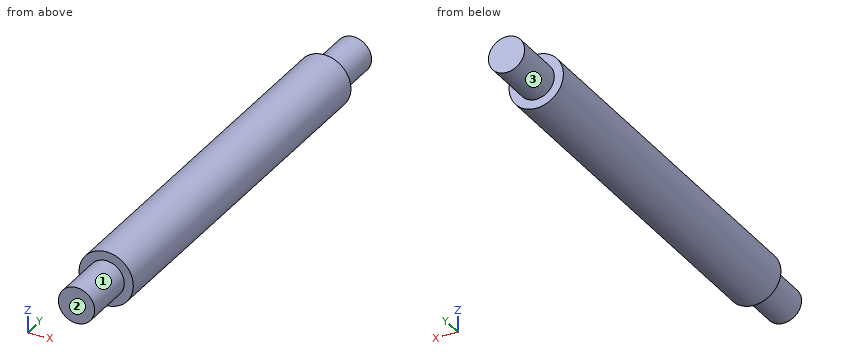
```python
from build123d import *

# Parameters (mm, degrees)
F0_R     = 4.7625
F1_DEPTH = 44.45
F2_R     = 6.35
F2_R_2   = 3.175
F3_DEPTH = 9.525
F4_R     = 6.35
F4_R_2   = 3.175
F5_DEPTH = 9.525


with BuildPart() as f1:
    # F0 (on Front) → F1 (new body, symmetric)
    with BuildSketch(Plane.XZ):
        Circle(F0_R)
    extrude(amount=F1_DEPTH, both=True)

    # F2 (on face) → F3 (cut)
    with BuildSketch(Plane.XZ.offset(44.45)):
        Circle(F2_R)
        Circle(F2_R_2, mode=Mode.SUBTRACT)
    extrude(amount=-F3_DEPTH, mode=Mode.SUBTRACT)

    # F4 (on face) → F5 (cut)
    with BuildSketch(Plane(origin=(0, 44.45, 0), x_dir=(-1, 0, 0), z_dir=(0, 1, 0))):
        Circle(F4_R)
        Circle(F4_R_2, mode=Mode.SUBTRACT)
    extrude(amount=-F5_DEPTH, mode=Mode.SUBTRACT)


solid = f1.part
```
Geometry: final body of the model. Coordinates: model frame, mm. Face numbers are marked on the shaded views. A direction names the side the tool comes from. Coordinates: 2 decimals unless noted, no trailing zeros. Order: outer loops, then holes, each group sorted by start corner. A loop starts at its lowest first (then second) coordinate and runs counter-clockwise, first axis right, second up. Notation, with made-up numbers: M 47.5,42 L 97.5,42 A12 cw 97.5,51 Z; hole C 36.25,-35.5 d6. An arc over 180 degrees is marked long. Answer as CSV lines item,"result".
Q1. Line query: probe 1 along Y at (x, z) = (-3.5, 1.75) (3 decimals); probe 2 along Z at (x, y) = (-0.25, 4); probe 3 along X at (y, z) = (-38.5, 2.25). Output: solid intervals per line, ascending. Write a range as [from, to].
Answers:
probe 1,"y = [-34.925, 34.925]"
probe 2,"z = [-4.76, 4.76]"
probe 3,"x = [-2.24, 2.24]"
Q2. Section D-D on x = 4. Return the cut outline in (y, z) (3 decimals), and give its area (3 significant figures).
Answers:
outline,"M -34.925,-2.585 L 34.925,-2.585 L 34.925,2.585 L -34.925,2.585 Z"
area,"361 mm^2"
Q3. Set-up query: the marked faces 1, 2 and 3. Return all of +Z, -Z, +X, -X, +Y, -Y with unobstructed straight access to the full face (end or side cutting, diameter ignored); none if empty.
Answers:
face 1,"-Y"
face 2,"+Z, -Z, +X, -X, -Y"
face 3,"+Y"
Q4. Section C-C on y = 21.5. Return the cut outline in (x, z) (1 decimal).
Answers:
outline,"C 0,0 d9.5"
Q5. First-contact query: P1, Ø2, axis at x = -3, y = -13.5, coming from the -Z side. Flat tip, straight axial feed; report the tip coordinate or a pass-through.
Answers:
P1,"stops at z = -4.32"
